For this review, take the finished solid that the model builds, in its own axes (mm). A direction names the side the tool comes from. Round coordinates to 2 decimals unless told otherwise and drop trailing zeros. Write each loop counter-clockwise with the first axis right and the second up, starting at its lowest first coordinate (ties: lowest second). Pieces come first, ordered by that corner, then holes. Notation, with made-up numbers: (-22.5, 43) - (10.5, 43) arc R26 cw to (10.5, 57) - close; hole circle Ø5 at (58.25, 11). An arc over 180 degrees is marked (long way). Answer in a Markdown table with one row per item. Add a question column.
from build123d import *

# Parameters (mm, degrees)
BOSS_EXTRUDE1_DEPTH = 2
BOSS_EXTRUDE2_DEPTH = 8
SKETCH5_R           = 1.5
CUT_EXTRUDE1_DEPTH  = 2
SKETCH6_R           = 1.5
CUT_EXTRUDE2_DEPTH  = 1.5


with BuildPart() as part:
    # Sketch1 → Boss-Extrude1 (new body)
    with BuildSketch(Plane.XY):
        with BuildLine():
            Line((-20, 32.5), (-9.993180492, 32.5))
            ThreePointArc((-9.993180492, 32.5), (0, 22.869247409), (9.993180492, 32.5))
            Line((9.993180492, 32.5), (20, 32.5))
            Line((20, 32.5), (20, -32.5))
            Line((20, -32.5), (-20, -32.5))
            Line((-20, -32.5), (-20, 32.5))
        make_face()
        with BuildLine():
            Line((-6.5, 17.5), (-6.5, -22.5))
            ThreePointArc((-6.5, -22.5), (-8, -24), (-9.5, -22.5))
            Line((-9.5, -22.5), (-9.5, 17.5))
            ThreePointArc((-9.5, 17.5), (-8, 19), (-6.5, 17.5))
        make_face(mode=Mode.SUBTRACT)
        with BuildLine():
            Line((6.5, 17.5), (6.5, -22.5))
            ThreePointArc((6.5, -22.5), (8, -24), (9.5, -22.5))
            Line((9.5, -22.5), (9.5, 17.5))
            ThreePointArc((9.5, 17.5), (8, 19), (6.5, 17.5))
        make_face(mode=Mode.SUBTRACT)
    extrude(amount=BOSS_EXTRUDE1_DEPTH)

    # Sketch2 → Boss-Extrude2 (add)
    with BuildSketch(Plane.XY.offset(2)):
        with BuildLine():
            Line((-20, 32.5), (-9.993180492, 32.5))
            ThreePointArc((-9.993180492, 32.5), (-9.904839947, 31.492967776), (-9.715280064, 30.5))
            Line((-9.715280064, 30.5), (-18.2, 30.5))
            Line((-18.2, 30.5), (-18.2, -30.5))
            Line((-18.2, -30.5), (18.2, -30.5))
            Line((18.2, -30.5), (18.2, 30.5))
            Line((18.2, 30.5), (9.715280064, 30.5))
            ThreePointArc((9.715280064, 30.5), (9.904839947, 31.492967776), (9.993180492, 32.5))
            Line((9.993180492, 32.5), (20, 32.5))
            Line((20, 32.5), (20, 30.5))
            Line((20, 30.5), (20, -30.5))
            Line((20, -30.5), (20, -32.5))
            Line((20, -32.5), (-20, -32.5))
            Line((-20, -32.5), (-20, -30.5))
            Line((-20, -30.5), (-20, 30.5))
            Line((-20, 30.5), (-20, 32.5))
        make_face()
    extrude(amount=BOSS_EXTRUDE2_DEPTH)

    # Sketch5 → Cut-Extrude1 (cut)
    with BuildSketch(Plane(origin=(0, 32.5, 0), x_dir=(1, 0, 0), z_dir=(0, 1, 0))):
        with Locations(Location((-15.5, -6.5, 0), (0, 0, 270))):
            Circle(SKETCH5_R)
        with Locations(Location((15.5, -6.5, 0), (0, 0, 90))):
            Circle(SKETCH5_R)
    extrude(amount=-CUT_EXTRUDE1_DEPTH, mode=Mode.SUBTRACT)

    # Sketch6 → Cut-Extrude2 (cut)
    with BuildSketch(Plane(origin=(0, -30.5, 0), x_dir=(1, 0, 0), z_dir=(0, 1, 0))):
        with Locations(Location((-15.5, -6.5, 0), (0, 0, 270))):
            Circle(SKETCH6_R)
        with Locations(Location((15.5, -6.5, 0), (0, 0, 90))):
            Circle(SKETCH6_R)
    extrude(amount=-CUT_EXTRUDE2_DEPTH, mode=Mode.SUBTRACT)


solid = part.part
Q1. Draft analysis for pull direction Y (two halves, no side actions). For faces 1 (the face through (0, -32.5, 5)), 2 (the face through (0, 0, 0)), 3 (the face through (13, 30.5, 6)), state which applies: released by +Y, released by -Y, zero draft, split by the parting line, or undercut.
Q2. Add section A-A on z = 6.5. State the section outline as (x, y) points, then the cut area to 3 significant figures.
Q3. Add section C-C on x = 13. State the section outline as (y, z) points.
Q4. Insertion check: pin 1 Ø8 at (x, y) = (-8, -9) entering from +Z; pin 2 Ø2.5 at (x, z) = (2, 7.5) entering from +Y; pin 3 Ø0.9 at (x, z) = (-15, 6.5) entering from +Y. Each pin has a flat end and moves straight along its axis. Give the tip position at first contact, or say it passes through.
Q5. Tool access review of faces 4 (the face through (-15, -32, 6)), 5 (the face through (18.2, 0, 6)), 6 (the face through (-8, -24, 1)): name each direction out of +Z, -Z, +X, -X, +Y, -Y from which nothing blocks a thin tool from reaching the whole face with its end or side.
Q6. Add section B-B on y = -17. State the section outline as (x, z) points, then the cut area to 3 significant figures.
Q7. To check wall thickness, follow probe 1 along X at (y, z) = (-14.5, 1.25); probe 2 along Z at (x, y) = (15.5, 31.2); probe 3 along Y at (x, z) = (10.5, 4). State the ranges of each line that lie inside material, in increasing order.
Q8. Add section D-D on x = 8. State the section outline as (y, z) points.
Answer sheet:
| question | item | result |
|---|---|---|
| 1 | face 1 | released by -Y |
| 1 | face 2 | zero draft |
| 1 | face 3 | undercut |
| 2 | outline | (-20, -32.5) - (20, -32.5) - (20, 32.5) - (17, 32.5) - (17, 30.5) - (18.2, 30.5) - (18.2, -30.5) - (17, -30.5) - (17, -32) - (14, -32) - (14, -30.5) - (-14, -30.5) - (-14, -32) - (-17, -32) - (-17, -30.5) - (-18.2, -30.5) - (-18.2, 30.5) - (-17, 30.5) - (-17, 32.5) - (-20, 32.5) - close; (-14, 30.5) - (-9.72, 30.5) arc R10 cw to (-9.99, 32.5) - (-14, 32.5) - close; (9.72, 30.5) - (14, 30.5) - (14, 32.5) - (9.99, 32.5) arc R10 cw to start |
| 2 | area | 319 mm² |
| 3 | outline | (-32.5, 0) - (32.5, 0) - (32.5, 10) - (30.5, 10) - (30.5, 2) - (-30.5, 2) - (-30.5, 10) - (-32.5, 10) - close |
| 4 | pin 1 | stops at z = 2 |
| 4 | pin 2 | stops at y = -30.5 |
| 4 | pin 3 | stops at y = -32 |
| 5 | face 4 | +Y |
| 5 | face 5 | +Z |
| 5 | face 6 | +Z, -Z |
| 6 | outline | (-20, 0) - (-9.5, 0) - (-9.5, 2) - (-18.2, 2) - (-18.2, 10) - (-20, 10) - close; (-6.5, 0) - (6.5, 0) - (6.5, 2) - (-6.5, 2) - close; (9.5, 0) - (20, 0) - (20, 10) - (18.2, 10) - (18.2, 2) - (9.5, 2) - close |
| 6 | area | 96.8 mm² |
| 7 | probe 1 | x = -20 to -9.5, -6.5 to 6.5, 9.5 to 20 |
| 7 | probe 2 | z = 0 to 5, 8 to 10 |
| 7 | probe 3 | y = -32.5 to -30.5, 30.5 to 32.5 |
| 8 | outline | (-32.5, 0) - (-24, 0) - (-24, 2) - (-30.5, 2) - (-30.5, 10) - (-32.5, 10) - close; (19, 0) - (26.87, 0) - (26.87, 2) - (19, 2) - close |
